The listing builds one solid part. Answer for the finished solid, in the listing's coordinates (mm). Give positions to 0.01 mm unless a question says otherwise; leave off trailing zeros. Write each loop counter-clockwise with the first axis right and the second up, starting at its lowest first coordinate (ties: lowest second). Pieces come first, ordered by that corner, then holes. Notation, with made-up numbers: M 72,34.5 L 93,34.5 A27 ccw 93,61.5 Z; hole C -19,88 d9. An arc over 180 degrees is marked long. Return JSON: item names as keys, results as strings.
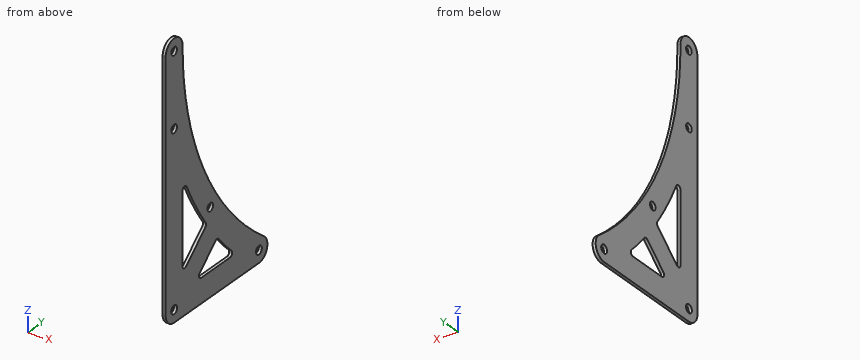
Autodesk Inventor part; units mm, degrees
ref_plane "YZ Plane" through (0, 0, 0) normal (1, 0, 0) x (0, 1, 0)
ref_plane "XZ Plane" through (0, 0, 0) normal (0, 1, 0) x (-1, 0, 0)
ref_plane "XY Plane" through (0, 0, 0) normal (0, 0, 1) x (1, 0, 0)
sketch "main" plane through (0, 0, 0) normal (0, 0, 1) x (1, 0, 0)
  circle A0 centre (-72.2021, -58.7899) radius 2.1844
  circle A1 centre (-8.7021, -58.7899) radius 2.1844
  circle A2 centre (-72.2021, 68.2101) radius 2.0955
  arc A3 (-65.8522, 68.1715) -> (-78.5521, 68.2101) centre (-72.2021, 68.2101) ccw
  arc A4 (-78.5521, -58.7899) -> (-72.2021, -65.1399) centre (-72.2021, -58.7899) ccw
  arc A5 (-8.7021, -65.1399) -> (-4.923, -53.6869) centre (-8.7021, -58.7899) ccw
  line L0 (-8.7021, -65.1399) -> (-72.2021, -65.1399)
  line L1 (-78.5521, -58.7899) -> (-78.5521, 68.2101)
  arc A6 (-65.8522, 68.1715) -> (-4.923, -53.6869) centre (84.6432, 67.2577) ccw
  circle A7 centre (-45.1241, -20.8434) radius 2.0955
  circle A8 centre (-72.2021, 30.1101) radius 2.0955
  line L2 (-30.2668, -52.4399) -> (-52.0453, -52.4399)
  line L3 (-65.8521, -40.4491) -> (-65.8521, -3.317)
  line L4 (-65.8521, 68.1906) -> (-65.8521, 68.2101)
  arc A9 (-30.2668, -52.4399) -> (-29.1598, -49.7146) centre (-30.2668, -50.8524) ccw
  arc A10 (-62.8301, -2.6371) -> (-65.8521, -3.317) centre (-64.2646, -3.317) ccw
  line L5 (-63.2196, -41.6442) -> (-48.8544, -29.0826)
  line L6 (-53.0903, -49.6574) -> (-41.1491, -39.2154)
  arc A11 (-62.8301, -2.6371) -> (-48.6032, -26.9709) centre (84.6432, 67.2577) ccw
  arc A12 (-38.9023, -39.3732) -> (-29.1598, -49.7146) centre (84.6432, 67.2577) ccw
  arc A13 (-48.8544, -29.0826) -> (-48.6032, -26.9709) centre (-49.8994, -27.8875) ccw
  arc A14 (-65.8521, -40.4491) -> (-63.2196, -41.6442) centre (-64.2646, -40.4491) ccw
  arc A15 (-53.0903, -49.6574) -> (-52.0453, -52.4399) centre (-52.0453, -50.8524) ccw
  arc A16 (-38.9023, -39.3732) -> (-41.1491, -39.2154) centre (-40.1041, -40.4105) ccw
  point P0 (-46.4652, -14.2849)
  point P1 (-26.2898, -52.4399)
  point P2 (-65.8521, 4.1323)
  point P3 (-47.7717, -28.1358)
  point P4 (-39.9404, -38.1585)
  point P5 (-65.3871, -51.9749)
  dimension "d0" = 4.191
  dimension "d1" = 12.7
  dimension "d3" = 4.191
  dimension "d4" = 4.191
  dimension "d8" = 1.5875
  dimension "d9" = 12.7
  dimension "d10" = 6.35
  dimension "d11" = 1.5875
sketch "Sketch1" plane through (0, 0, 0) normal (1, 0, 0) x (0, 1, 0)
  circle A0 centre (0, 0) radius 2.1844
  circle A1 centre (63.5, 0) radius 2.1844
  circle A2 centre (0, 127) radius 2.0955
  arc A3 (6.3499, 126.9614) -> (-6.35, 127) centre (0, 127) ccw
  arc A4 (-6.35, 0) -> (0, -6.35) centre (0, 0) ccw
  arc A5 (63.5, -6.35) -> (67.2791, 5.103) centre (63.5, 0) ccw
  line L0 (63.5, -6.35) -> (0, -6.35)
  line L1 (-6.35, 0) -> (-6.35, 127)
  arc A6 (6.3499, 126.9614) -> (67.2791, 5.103) centre (156.8453, 126.0476) ccw
  circle A7 centre (27.078, 37.9465) radius 2.0955
  circle A8 centre (0, 88.9) radius 2.0955
  line L2 (41.9353, 6.35) -> (20.1568, 6.35)
  line L3 (6.35, 18.3408) -> (6.35, 55.4729)
  line L4 (6.35, 126.9805) -> (6.35, 127)
  arc A9 (41.9353, 6.35) -> (43.0423, 9.0753) centre (41.9353, 7.9375) ccw
  arc A10 (9.372, 56.1528) -> (6.35, 55.4729) centre (7.9375, 55.4729) ccw
  line L5 (8.9825, 17.1457) -> (23.3477, 29.7074)
  line L6 (19.1118, 9.1325) -> (31.053, 19.5745)
  arc A11 (9.372, 56.1528) -> (23.5989, 31.819) centre (156.8453, 126.0476) ccw
  arc A12 (33.2998, 19.4167) -> (43.0423, 9.0753) centre (156.8453, 126.0476) ccw
  arc A13 (23.3477, 29.7074) -> (23.5989, 31.819) centre (22.3027, 30.9024) ccw
  arc A14 (6.35, 18.3408) -> (8.9825, 17.1457) centre (7.9375, 18.3408) ccw
  arc A15 (19.1118, 9.1325) -> (20.1568, 6.35) centre (20.1568, 7.9375) ccw
  arc A16 (33.2998, 19.4167) -> (31.053, 19.5745) centre (32.098, 18.3794) ccw
extrude "Extrusion1" add sketch "Sketch1" against normal blind 1.5875
properties part number "Scoop Gusset" material "Acetal Resin, White"
Item 1: A cutting plane is placed at D-D, the plane z = 68. Write down the section's boundary in (x, y), plus the area to 3 significant figures.
Geometry results:
{"outline": "M -1.59,-6.35 L 0,-6.35 L 0,17.99 L -1.59,17.99 Z", "area": "38.6 mm2"}
Item 2: A cutting plane is placed at A-A, the plane x = -0.4. Count the separate pieces of the cut face and the enclosed holes in it, plus the area to 3 significant figures.
Geometry results:
{"separate pieces": "1", "enclosed holes": "7", "area": "4,010 mm2"}
Item 3: Find the intervals of material crossed by line 1 (Z direction, x = -0.45, y = 0); line 2 (Z direction, x = -0.2, y = 28.5); line 3 (Z direction, x = -1.1, y = 22.5), in increasing order.
Geometry results:
{"line 1": "z = -6.35 to -2.18, 2.18 to 86.8, 91 to 124.9, 129.1 to 133.35", "line 2": "z = -6.35 to 6.35, 17.34 to 36.41, 39.49 to 47.45", "line 3": "z = -6.35 to 6.35, 12.1 to 28.97, 33.39 to 58.22"}
Item 4: A cutting plane is placed at C-C, the plane y = 5. Write down the section's boundary in (x, z).
Geometry results:
{"outline": "M -1.59,-6.35 L 0,-6.35 L 0,130.91 L -1.59,130.91 Z"}
Item 5: Given pin 1 Ø2 at (y, z) = (3, 64) entering from +X, flat-ended and moving along its own axis, determine where the tip first touches the part or whether it passes through.
Geometry results:
{"pin 1": "stops at x = 0"}
Item 6: A cutting plane is placed at B-B, the plane z = 88.9. Write down the section's boundary in (x, y).
Geometry results:
{"outline": "M -1.59,-6.35 L 0,-6.35 L 0,-2.1 L -1.59,-2.1 Z; M -1.59,2.1 L 0,2.1 L 0,11 L -1.59,11 Z"}
